Autodesk Inventor part; units mm, degrees
ref_plane "YZ Plane" through (0, 0, 0) normal (1, 0, 0) x (0, 1, 0)
ref_plane "XZ Plane" through (0, 0, 0) normal (0, 1, 0) x (-1, 0, 0)
ref_plane "XY Plane" through (0, 0, 0) normal (0, 0, 1) x (1, 0, 0)
sketch "Sketch1" plane through (0, 0, 0) normal (0, 1, 0) x (-1, 0, 0)
  circle A0 centre (0, 0) radius 6
  dimension "d0" = 12
extrude "srodek" add sketch "Sketch1" along normal blind 6
sketch "Sketch2" plane through (0, 0, 0) normal (0, -1, 0) x (1, 0, 0)
  circle A0 centre (0, 0) radius 6
  circle A1 centre (0, 0) radius 3
  dimension "d3" = 6
extrude "dolne" add sketch "Sketch2" along normal blind 10 contours A1
thread "Thread1"
chamfer "Chamfer1" distance 0.5 angle 45 1 edges at (-3, -10, 0)
sketch "Sketch3" plane through (0, 0, 0) normal (0, 0, 1) x (1, 0, 0)
  line L0 (3, 0) -> (-3, 0)
  line L1 (-3, 0) -> (-2.5, 0)
  line L2 (-2.5, 0) -> (-2.5, -0.5)
  line L3 (-2.5, -0.5) -> (-3, -0.5)
  line L4 (-3, -0.5) -> (-3, 0)
  line L5 (0, -0.6) -> (0, 0.1)
  point P0 (0, 0)
  point P1 (-2.5, 0)
  dimension "d11" = 0.5
  dimension "d12" = 0.5
revolve "Revolution1" cut sketch "Sketch3" angle 360 about axis through (0, -10, 0) along (0, 1, 0)
sketch "Sketch6" plane through (0, 6, 0) normal (0, 1, 0) x (1, 0, 0)
  circle A0 centre (0, 0) radius 4
  circle A1 centre (0, 0) radius 3
  dimension "d19" = 6
extrude "mocowanie K1" add sketch "Sketch6" along normal blind 10 contours A1
sketch "Sketch7" plane through (0, 0, 0) normal (1, 0, 0) x (0, 1, 0)
  line L0 (6, -3) -> (6.5, -3)
  line L1 (6.5, -3) -> (6.5, -2.5)
  line L2 (6.5, -2.5) -> (6, -2.5)
  line L3 (6, -2.5) -> (6, -3)
  line L4 (-3.2, 0) -> (19.2, 0)
  line L5 (16, -3) -> (16, 3) construction
  line L6 (6, 3) -> (6, -3) construction
  point P0 (0, 0)
  dimension "d27" = 0.5
  dimension "d28" = 0.5
revolve "Revolution2" cut sketch "Sketch7" angle 360 about axis through (0, -10, 0) along (0, 1, 0)
thread "Thread3"
chamfer "Chamfer3" distance 0.5 angle 45 1 edges at (-3, 16, 0)
properties part number "KN-00-02-04" material "X5CrNi18-10"
Work out the finished part from the listing and answer in its coordinate system (mm). A direction names the side the tool comes from. Give positions to 0.01 mm unless a question says otherwise; leave off trailing zeros. Loops run counter-clockwise (first coordinate to the right, second up) from the corner with the lowest first, then second, coordinate; pieces in that order, holes last. Notation, with made-up numbers: (-21.5, 72.25) -> (-11.5, 72.25) arc R21 ccw to (-11.5, 77.25) -> close; hole circle Ø8 at (28.5, -13.75). An arc over 180 degrees is marked (long way). One line per question, with ' | ' between items. Start each with the question number.
1) Section A-A, the plane z = 0 is taken. Determine the outline of the cut face in (x, y), then the cut area to 4 significant figures.
2) Each of these flat-tipped pins is pushed along its axis until it touches: pin 1 (2 mm diameter, centred on y = 3, z = 3.5, fed in from -X); pin 2 (1.5 mm diameter, centred on y = -1, z = 1, fed in from -X); pin 3 (5 mm diameter, centred on x = -4, y = 10.5, fed in from -Z). Where does it stop, or does it pass through?
3) Straight lines are drawn through the part: L1, parallel to Y at x = 2.25, z = -3.5; L2, parallel to X at y = -1.25, z = 0; L3, parallel to X at y = 7, z = 2. For each, find the intervals that lie inside material, in ascending order.
4) For faces 5 (the face through (-3, 11, 0)), 6 (the face through (-2.44, 6.25, 0.54)), 7 (the face through (0, 16, 0)), 8 (the face through (-3, -5, 0)), determine the directions among +Z, -Z, +X, -X, +Y, -Y from which every point of the face is accessible in a straight line to the end or side of a thin tool.
5) Section C-C, the plane y = -1.75 is taken. Determine the outline of the cut face in (x, z), then the cut area to 3 significant figures.
6) Section D-D, the plane x = -5 is taken. Determine the outline of the cut face in (y, z).
7) Determine the mould class of faces 1 (the face through (-2, 6.5, 2)), 2 (the face through (0.54, -0.25, 2.44)), 3 (the face through (6, 3, 0)), 4 (the face through (0, -10, 0)) for opening direction Y: +Y half, -Y half, draft (parallel to the pull), parting line (faces both ways), or undercut.
8) Section B-B, the plane x = 0 is taken. Determine the outline of the cut face in (y, z), then the cut area to 4 significant figures.
Resolved:
1) outline: (-6, 0) -> (-2.5, 0) -> (-2.5, -0.5) -> (-3, -0.5) -> (-3, -9.5) -> (-2.5, -10) -> (2.5, -10) -> (3, -9.5) -> (3, -0.5) -> (2.5, -0.5) -> (2.5, 0) -> (6, 0) -> (6, 6) -> (2.5, 6) -> (2.5, 6.5) -> (3, 6.5) -> (3, 15.5) -> (2.5, 16) -> (-2.5, 16) -> (-3, 15.5) -> (-3, 6.5) -> (-2.5, 6.5) -> (-2.5, 6) -> (-6, 6) -> close | area: 190.5 mm2
2) pin 1: x = -5.45 | pin 2: x = -2.99 | pin 3: z = -2.6
3) L1: 0 to 6 | L2: -3 to 3 | L3: -2.24 to 2.24
4) face 5: +Y | face 6: none | face 7: +Z, -Z, +X, -X, +Y | face 8: -Y
5) outline: circle Ø6 at (0, 0) | area: 28.3 mm2
6) outline: (0, -3.32) -> (6, -3.32) -> (6, 3.32) -> (0, 3.32) -> close
7) face 1: undercut | face 2: undercut | face 3: draft | face 4: -Y half
8) outline: (-10, -2.5) -> (-9.5, -3) -> (-0.5, -3) -> (-0.5, -2.5) -> (0, -2.5) -> (0, -6) -> (6, -6) -> (6, -2.5) -> (6.5, -2.5) -> (6.5, -3) -> (15.5, -3) -> (16, -2.5) -> (16, 2.5) -> (15.5, 3) -> (6.5, 3) -> (6.5, 2.5) -> (6, 2.5) -> (6, 6) -> (0, 6) -> (0, 2.5) -> (-0.5, 2.5) -> (-0.5, 3) -> (-9.5, 3) -> (-10, 2.5) -> close | area: 190.5 mm2
